Autodesk Inventor part; units mm, degrees
ref_plane "to_screw1_XY" through (12, 0, 6.8) normal (0, 0, 1) x (1, 0, 0)
ref_plane "to_screw1_YZ" through (12, 0, 6.8) normal (1, 0, 0) x (0, 1, 0)
ref_plane "to_screw1_ZX" through (12, 0, 6.8) normal (0, 1, 0) x (0, 0, 1)
sketch "Sketch_1" plane through (0, 0, 0) normal (0, 0, 1) x (1, 0, 0)
  line L0 (20, 0) -> (0, 0)
  line L1 (0, 5) -> (20, 5)
  line L2 (20, 5) -> (20, 10)
  line L3 (20, 10) -> (5, 10)
  line L4 (5, 10) -> (5, 19)
  line L5 (5, 19) -> (0, 19)
  line L6 (0, 19) -> (0, 5)
revolve "Revolution1" add sketch "Sketch_1" angle 360 about axis through (20, 0, 0) along (1, 0, 0)
sketch "Sketch2" plane through (0, 0, 0) normal (-1, 0, 0) x (0, 0, 1)
  point P0 (-10.6066, 10.6066)
hole "Hole1" at (0, 10.6066, -10.6066) direction (1, 0, 0) diameter 3.5 depth 5
pattern_linear "Rectangular Pattern1" count 2 spacing 21.2132 along (0, 0, 1) count 2 spacing 21.2132 along (0, -1, 0) of "Hole1"
sketch "Sketch_4" plane through (12, 0, 0) normal (1, 0, 0) x (0, 0, -1)
  line L0 (0, -10) -> (0, -4)
  line L1 (0, -4) -> (1.2295, -4)
  line L2 (1.2295, -4) -> (1.2295, -9.7295)
  line L3 (1.2295, -9.7295) -> (1.5, -10)
  line L4 (1.5, -10) -> (0, -10)
  line L5 (0, -10) -> (0, -4)
revolve "Revolution2" cut sketch "Sketch_4" angle 360 about axis through (12, -10, 0) along (0, -1, 0)
thread "Thread1"
sketch "Sketch_8" plane through (0, 0, 0) normal (1, 0, 0) x (0, 1, 0)
  line L0 (1.5, 6.8) -> (-1.5, 6.8)
  line L1 (-1.5, 6.8) -> (-1.5, 0)
  line L2 (-1.5, 0) -> (1.5, 0)
  line L3 (1.5, 0) -> (1.5, 6.8)
extrude "Extrusion1" cut sketch "Sketch_8" along normal blind 20
sketch "Sketch_5" plane through (12, 0, 0) normal (1, 0, 0) x (0, 0, -1)
  line L0 (-5, 0) -> (-10, 0)
  line L1 (-10, 0) -> (-10, 1.5)
  line L2 (-10, 1.5) -> (-9.7295, 1.2295)
  line L3 (-9.7295, 1.2295) -> (-5, 1.2295)
  line L4 (-5, 1.2295) -> (-5, 0)
  line L5 (-5, 0) -> (-10, 0)
revolve "Revolution3" cut sketch "Sketch_5" angle 360 about axis through (12, 0, 5) along (0, 0, -1)
thread "Thread2"
ref_plane "to_screw1_XY" through (12, 0, 6.8) normal (0, 0, 1) x (1, 0, 0)
ref_plane "to_screw1_YZ" through (12, 0, 6.8) normal (1, 0, 0) x (0, 1, 0)
ref_plane "to_screw1_ZX" through (12, 0, 6.8) normal (0, 1, 0) x (0, 0, 1)
ref_plane "to_screw2_XY" through (12, -5, 0) normal (0, -1, 0) x (1, 0, 0)
ref_plane "to_screw2_YZ" through (12, -5, 0) normal (1, 0, 0) x (0, 0, 1)
ref_plane "to_screw2_ZX" through (12, -5, 0) normal (0, 0, 1) x (0, -1, 0)
properties part number "STHRANG10-MB_ss"
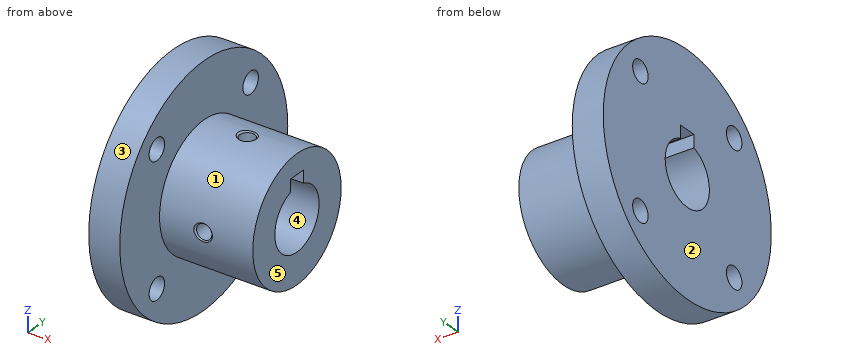
CAD build for the part. Positions are in the model's coordinates, mm. Face numbers are marked on the shaded views. A direction names the side the tool comes from. Coordinates: 2 decimals unless noted, no trailing zeros. Order: outer loops, then holes, each group sorted by start corner. A loop starts at its lowest first (then second) coordinate and runs counter-clockwise, first axis right, second up. Notation, with made-up numbers: (57, 13) - (73, 13) arc R25 cw to (73, 50) - close; hole circle Ø1 at (35, 45.25). An arc over 180 degrees is marked (long way). Use a Markdown table: item, result. Add a question column.
(1) Flat gauge pins, fed straight in: pin 1 (3 mm diameter, centred on x = 3, y = -13, fed in from +Z); pin 2 (2 mm diameter, centred on x = 13.5, z = 6, fed in from +Y); pin 3 (3 mm diameter, centred on y = -10.61, z = 10.61, fed in from +X); pin 4 (3.5 mm diameter, centred on x = 10.5, y = -0.5, fed in from -Z). Where does each tip first touch, or does it go through?
(2) Pull direction Z, two halves, no side cores. Call the marked faces 3, 4 and 5: +Z half, -Z half, draft (parallel to the pull), parting line (faces both ways), or undercut.
(3) Saw through at C-C (x = 12). Give the cut face in (y, z), then the cut area to 3 significant figures.
(4) Saw through at A-A (z = 0). Give the cut face in (x, y), then the cut area to 3 significant figures.
(5) Saw through at D-D (x = 6.75). Give the cut face in (y, z), then the cut area to 3 significant figures.
(6) Which spindle directions (+Z, -Z, +X, -X, +Y, -Y) get a long thin tool onto all of the face, cutting with end or side? Do the marked faces 1 and 2. Say none if no direction does.
(7) Drill centre lines: line 1 along Z through (x, y) = (15.5, 0); line 2 along X through (y, z) = (-7.6, 0); line 3 along X through (y, z) = (2, 14). Where is each one in solid material? Low to high. Write a range as [from, to].
(8) Saw through at B-B (y = 0). Give the cut face in (x, z).
Solved:
| question | item | result |
|---|---|---|
| 1 | pin 1 | stops at z = 15.12 |
| 1 | pin 2 | stops at y = 8.66 |
| 1 | pin 3 | passes through |
| 1 | pin 4 | stops at z = -10 |
| 2 | face 3 | parting line |
| 2 | face 4 | undercut |
| 2 | face 5 | draft |
| 3 | outline | (-9.9, -1.4) arc R10 ccw (long way) to (1.4, 9.9) - (1.23, 9.73) - (1.23, 6.8) - (1.5, 6.8) - (1.5, 4.77) arc R5 cw (long way) to (-4.85, -1.23) - (-9.73, -1.23) - close; (-9.9, 1.4) - (-9.73, 1.23) - (-4.85, 1.23) arc R5 cw to (-1.5, 4.77) - (-1.5, 6.8) - (-1.23, 6.8) - (-1.23, 9.73) - (-1.4, 9.9) arc R10 ccw to start |
| 3 | area | 210 mm² |
| 4 | outline | (0, -19) - (5, -19) - (5, -10) - (10.5, -10) - (10.77, -9.73) - (10.77, -5) - (0, -5) - close; (0, 5) - (20, 5) - (20, 10) - (5, 10) - (5, 19) - (0, 19) - close; (13.23, -9.73) - (13.5, -10) - (20, -10) - (20, -5) - (13.23, -5) - close |
| 4 | area | 278 mm² |
| 5 | outline | circle Ø20 at (0, 0); hole (-1.5, 4.77) arc R5 ccw (long way) to (1.5, 4.77) - (1.5, 6.8) - (-1.5, 6.8) - close |
| 5 | area | 230 mm² |
| 6 | face 1 | +X |
| 6 | face 2 | +Z, -Z, -X, +Y, -Y |
| 7 | line 1 | z = [-10, -5], [6.8, 10] |
| 7 | line 2 | x = [0, 10.77], [13.23, 20] |
| 7 | line 3 | x = [0, 5] |
| 8 | outline | (0, -19) - (5, -19) - (5, -10) - (20, -10) - (20, -5) - (0, -5) - close; (0, 6.8) - (10.77, 6.8) - (10.77, 9.73) - (10.5, 10) - (5, 10) - (5, 19) - (0, 19) - close; (13.23, 6.8) - (20, 6.8) - (20, 10) - (13.5, 10) - (13.23, 9.73) - close |
